Part model, mm, in its own coordinate system. A direction names the side the tool comes from. Give positions to 0.01 mm unless a question says otherwise; leave off trailing zeros. Order: outer loops, then holes, each group sorted by start corner. A loop starts at its lowest first (then second) coordinate and runs counter-clockwise, first axis right, second up. Notation, with made-up numbers: (56.25, 12) - (104.25, 12) arc R23 ccw to (104.25, 40) - close; hole circle Ø6 at (16, 9). An arc over 180 degrees is marked (long way). Use one line per item in the form item = value. Start each with the question number.
1. Drill centre lines: line 1 (Y direction, x = 32.5, z = 48); line 2 (Y direction, x = -18, z = 31.5). Where is each one in solid material? Low to high.
2. Band-saw the part on C-C, the plane y = 6.5. List the corners of the cut face in (x, z), plus the area to 3 significant figures.
3. Band-saw the part on B-B, the plane x = 5. List the corners of the cut face in (y, z).
4. Band-saw the part on A-A, the plane z = 68.5. List the corners of the cut face in (x, y), plus the area to 3 significant figures.
5. Tool access for faces 4 (the face through (0, 20, 1)), 5 (the face through (23, 0, 2.5)), 6 (the face through (0, -36, 7)), 7 (the face through (-36.232, 0.623, 66.987)), 8 (the face through (-1, 48, 55)): list every direction of +Z, -Z, +X, -X, +Y, -Y with a clear straight run to the whole face (end or side of a thin tool).
6. Pin check, flat tips, straight feed: P1, Ø1.2, axis at x = -5.5, z = 2, coming from the +Y side; P2, Ø3, axis at x = -3.5, y = 49.5, coming from the -Z side. Stop position of each tip, or through.
7. Band-saw the part on D-D, the plane x = -26. List the corners of the cut face in (y, z).
8. Pull direction X, two halves, no side cores. Call faces 1 (the face through (36.268, 0.623, 66.987)), 2 (the face through (-16, 35, 40)), 3 (the face through (-37.5, 19, 39)): +X half, -X half, draft (parallel to the pull), parting line (faces both ways), or undercut.
from build123d import *

# Parameters (mm, degrees)
F0_W      = 75
F0_H      = 75
F0_W_2    = 70
F0_H_2    = 70
F1_DEPTH  = 80
F2_T      = -2.5
F4_DEPTH  = 75.001
F5_W      = 75
F5_H      = 40
F6_DEPTH  = 17
F7_W      = 75
F7_H      = 10.5
F8_DEPTH  = 30
F9_R      = 2
F11_DEPTH = 75.001
F13_DEPTH = 80.6
F15_DEPTH = 2.501


with BuildPart() as f1:
    # F0 (on Top) → F1 (new body)
    with BuildSketch(Plane.XY):
        Rectangle(F0_W, F0_H)
        Rectangle(F0_W_2, F0_H_2, mode=Mode.SUBTRACT)
        Rectangle(F0_W_2, F0_H_2)
    extrude(amount=F1_DEPTH)

    # F2
    f2_openings = [f1.faces().sort_by_distance(p)[0] for p in [
        (0, 0, 80),
    ]]
    offset(amount=F2_T, openings=f2_openings)

    # F3 (on face) → F4 (cut, through all)
    with BuildSketch(Plane(origin=(-37.5, 0, 0), x_dir=(0, -1, 0), z_dir=(-1, 0, 0))):
        Polygon((37.5, 80), (-32.6899588108, 80), (37.5, 69.7793290019), align=None)
    extrude(amount=-F4_DEPTH, mode=Mode.SUBTRACT)

    # F5 (on face) → F6 (join)
    with BuildSketch(Plane(origin=(0, 37.5, 0), x_dir=(-1, 0, 0), z_dir=(0, 1, 0))):
        with Locations((0, 60)):
            Rectangle(F5_W, F5_H)
    extrude(amount=F6_DEPTH)

    # F7 (on face) → F8 (cut)
    with BuildSketch(Plane(origin=(0, 0, 40), x_dir=(1, 0, 0), z_dir=(0, 0, -1))):
        with Locations((0, -42.75)):
            Rectangle(F7_W, F7_H)
    extrude(amount=-F8_DEPTH, mode=Mode.SUBTRACT)

    # F9
    f9_edges = [f1.edges().sort_by_distance(p)[0] for p in [
        (0, 54.5, 80),
        (-37.5, -37.5, 34.889665),
        (37.5, -37.5, 34.889665),
        (0, 35, 80),
    ]]
    fillet(f9_edges, radius=F9_R)

    # F10 (on face) → F11 (cut, through all)
    with BuildSketch(Plane.YZ.offset(37.5)):
        with BuildLine():
            Line((-14.9888207723, 52.579009374), (-14.998647473, 21.7985701573))
            ThreePointArc((-14.998647473, 21.7985701573), (0.2893425083, 7.0027908959), (14.9952554508, 22.3772452324))
            Line((14.9952554508, 22.3772452324), (14.9999923512, 51.9848519034))
            ThreePointArc((14.9999923512, 51.9848519034), (0.2971312437, 66.9970568121), (-14.9888207723, 52.579009374))
        make_face()
    extrude(amount=-F11_DEPTH, mode=Mode.SUBTRACT)

    # F12 (on face) → F13 (cut)
    with BuildSketch(Plane.XZ.offset(37.5)):
        with BuildLine():
            Line((-14.9889976507, 47.5744122453), (-14.9999986115, 22.0064539529))
            ThreePointArc((-14.9999986115, 22.0064539529), (0.0022397735, 7.0000001672), (14.9999960153, 22.0109334991))
            Line((14.9999960153, 22.0109334991), (14.9812347551, 47.7500701389))
            ThreePointArc((14.9812347551, 47.7500701389), (-0.0879146719, 61.9997423648), (-14.9889976507, 47.5744122453))
        make_face()
    extrude(amount=-F13_DEPTH, mode=Mode.SUBTRACT)

    # F14 (on face) → F15 (cut, through all)
    with BuildSketch(Plane.XY.offset(2.5)):
        with BuildLine():
            Line((15, 20), (-15, 20))
            ThreePointArc((-15, 20), (-18.5355339059, 18.5355339059), (-20, 15))
            Line((-20, 15), (-20, -15))
            ThreePointArc((-20, -15), (-18.5355339059, -18.5355339059), (-15, -20))
            Line((-15, -20), (15, -20))
            ThreePointArc((15, -20), (18.5355339059, -18.5355339059), (20, -15))
            Line((20, -15), (20, 15))
            ThreePointArc((20, 15), (18.5355339059, 18.5355339059), (15, 20))
        make_face()
    extrude(amount=-F15_DEPTH, mode=Mode.SUBTRACT)


solid = f1.part
From the geometry:
q1.line_1 = -37.5 to -35, 35 to 37.5, 48 to 54.5
q1.line_2 = -37.5 to -35, 35 to 37.5
q2.outline = (-37.5, 0) - (-20, 0) - (-20, 2.5) - (-35, 2.5) - (-35, 8.48) - (-37.5, 8.48) - close; (-37.5, 65.52) - (-35, 65.52) - (-35, 76.19) - (-37.5, 76.19) - close; (20, 0) - (37.5, 0) - (37.5, 8.48) - (35, 8.48) - (35, 2.5) - (20, 2.5) - close; (35, 65.52) - (37.5, 65.52) - (37.5, 76.19) - (35, 76.19) - close
q2.area = 171 mm²
q3.outline = (-37.5, 0) - (-20, 0) - (-20, 2.5) - (-35, 2.5) - (-35, 7.86) - (-37.5, 7.86) - close; (-37.5, 61.14) - (-35, 61.14) - (-35, 70.14) - (-37.5, 69.78) - close; (20, 0) - (37.5, 0) - (37.5, 7.86) - (35, 7.86) - (35, 2.5) - (20, 2.5) - close; (35, 61.14) - (37.5, 61.14) - (37.5, 70) - (48, 70) - (48, 40) - (54.5, 40) - (54.5, 78) arc R2 ccw to (52.5, 80) - (37, 80) arc R2 ccw to (35, 78) - close
q4.outline = (-37.5, -35.5) arc R2 ccw to (-35.5, -37.5) - (35.5, -37.5) arc R2 ccw to (37.5, -35.5) - (37.5, 37.5) - (-37.5, 37.5) - close; (-37.5, 48) - (37.5, 48) - (37.5, 54.5) - (-37.5, 54.5) - close; hole (-35, -35) - (35, -35) - (35, 35) - (-35, 35) - close
q4.area = 1,210 mm²
q5.face_4 = +Z, -Z
q5.face_5 = +Z
q5.face_6 = +Y, -Y
q5.face_7 = +X, -X
q5.face_8 = -Z, +X, -X
q6.P1 = 37.5
q6.P2 = 40
q7.outline = (-37.5, 0) - (37.5, 0) - (37.5, 70) - (48, 70) - (48, 40) - (54.5, 40) - (54.5, 78) arc R2 ccw to (52.5, 80) - (37, 80) arc R2 ccw to (35, 78) - (35, 2.5) - (-35, 2.5) - (-35, 70.14) - (-37.5, 69.78) - close
q8.face_1 = draft
q8.face_2 = undercut
q8.face_3 = -X half
